```python
from build123d import *

# Parameters (mm, degrees)
F0_R     = 5.9319111077
F1_DEPTH = 114.3
F2_W     = 74.0328431129
F2_H     = 50.0019490719
F2_W_2   = 18.4651985765
F3_DEPTH = 30.2013677934
F4_DEPTH = 81.026


with BuildPart() as f1:
    # F0 (on Top) → F1 (new body)
    with BuildSketch(Plane.XY):
        with BuildLine():
            Line((15.1001838967, -37.0164215565), (15.1001838967, 37.0164215565))
            ThreePointArc((15.1001838967, 37.0164215565), (0, 21.9162376598), (-15.1001838967, 37.0164215565))
            Line((-15.1001838967, 37.0164215565), (-15.1001838967, -37.0164215565))
            ThreePointArc((-15.1001838967, -37.0164215565), (0, -21.9162376598), (15.1001838967, -37.0164215565))
        make_face()
        with BuildLine():
            ThreePointArc((-15.1001838967, -37.0164215565), (0, -52.1166054532), (15.1001838967, -37.0164215565))
            ThreePointArc((15.1001838967, -37.0164215565), (0, -21.9162376598), (-15.1001838967, -37.0164215565))
        make_face()
        with Locations((0, -37.0164215565)):
            Circle(F0_R, mode=Mode.SUBTRACT)
        with BuildLine():
            ThreePointArc((-15.1001838967, 37.0164215565), (0, 21.9162376598), (15.1001838967, 37.0164215565))
            ThreePointArc((15.1001838967, 37.0164215565), (0, 52.1166054532), (-15.1001838967, 37.0164215565))
        make_face()
        with Locations((0, 37.0164215565)):
            Circle(F0_R, mode=Mode.SUBTRACT)
    extrude(amount=F1_DEPTH)

    # F2 (on face) → F3 (cut, through all)
    with BuildSketch(Plane.YZ.offset(15.1001838967)):
        with Locations((0, 52.5265261531)):
            Rectangle(F2_W, F2_H)
        with Locations((-46.2490208447, 52.5265261531)):
            Rectangle(F2_W_2, F2_H)
        with Locations((46.2490208447, 52.5265261531)):
            Rectangle(F2_W_2, F2_H)
    extrude(amount=-F3_DEPTH, mode=Mode.SUBTRACT)

    # F0 (on Top) → F4 (join)
    with BuildSketch(Plane.XY):
        with BuildLine():
            ThreePointArc((-15.1001838967, 37.0164215565), (0, 21.9162376598), (15.1001838967, 37.0164215565))
            ThreePointArc((15.1001838967, 37.0164215565), (0, 52.1166054532), (-15.1001838967, 37.0164215565))
        make_face()
        with Locations((0, 37.0164215565)):
            Circle(F0_R, mode=Mode.SUBTRACT)
    extrude(amount=F4_DEPTH)


solid = f1.part
```
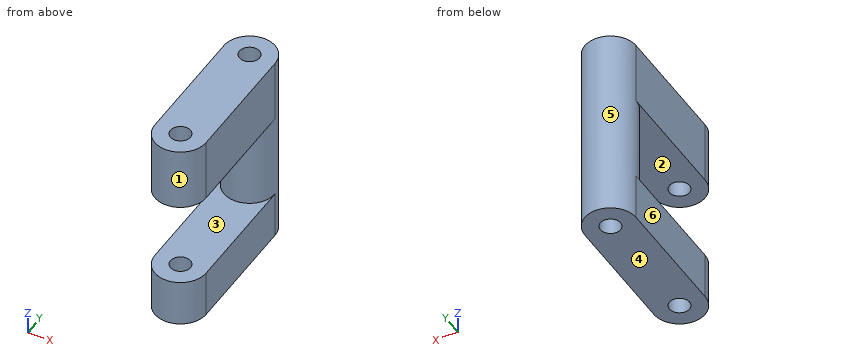
Build history of the part. All positions in model axes, mm. Face numbers are marked on the shaded views. A direction names the side the tool comes from. Give positions to 0.01 mm unless a question says otherwise; leave off trailing zeros. Loops run counter-clockwise (first coordinate to the right, second up) from the corner with the lowest first, then second, coordinate; pieces in that order, holes last.
Item 1: Slice it at A-A, the plane y = -6.5. List the corners of the cut face in (x, z).
Answers follow:
outline: (-15.1, 0) - (15.1, 0) - (15.1, 27.53) - (-15.1, 27.53) - close; (-15.1, 77.53) - (15.1, 77.53) - (15.1, 114.3) - (-15.1, 114.3) - close
Item 2: Which spindle directions (+Z, -Z, +X, -X, +Y, -Y) get a long thin tool onto all of the face, cutting with end or side? Do the marked faces 5 and 6. Say none if no direction does.
Answers follow:
face 5: none
face 6: +Z, -Z, -X, +Y, -Y
Item 3: Drill centre lines: line 1 (Y direction, x = 0, z = 19.75); line 2 (Y direction, x = 0, z = 37); line 3 (Z direction, x = -4, y = -9). Where is each one in solid material? Low to high.
Answers follow:
line 1: y = -52.12 to -42.95, -31.08 to 31.08, 42.95 to 52.12
line 2: y = 21.92 to 31.08, 42.95 to 52.12
line 3: z = 0 to 27.53, 77.53 to 114.3
Item 4: Slice it at D-D, the plane y = -45. List the corners of the cut face in (x, z).
Answers follow:
outline: (-12.82, 0) - (12.82, 0) - (12.82, 27.53) - (-12.82, 27.53) - close; (-12.82, 77.53) - (12.82, 77.53) - (12.82, 114.3) - (-12.82, 114.3) - close
Item 5: Slice it at B-B, the plane x = 0. List the corners of the cut face in (y, z).
Answers follow:
outline: (-52.12, 0) - (-42.95, 0) - (-42.95, 27.53) - (-52.12, 27.53) - close; (-52.12, 77.53) - (-42.95, 77.53) - (-42.95, 114.3) - (-52.12, 114.3) - close; (-31.08, 0) - (31.08, 0) - (31.08, 114.3) - (-31.08, 114.3) - (-31.08, 77.53) - (21.92, 77.53) - (21.92, 27.53) - (-31.08, 27.53) - close; (42.95, 0) - (52.12, 0) - (52.12, 114.3) - (42.95, 114.3) - close
Item 6: Flat gauge pins, fed straight in: pin 1 (10.5 mm diameter, centred on x = 0, y = 37.02, fed in from +Z); pin 2 (8 mm diameter, centred on y = -41.5, z = 98, fed in from -X); pin 3 (3 mm diameter, centred on x = -7.5, z = 16, fed in from +Y); pin 4 (6 mm diameter, centred on x = -9.5, z = 36, fed in from +Y). Where does each tip first touch, or does it go through?
Answers follow:
pin 1: passes through
pin 2: stops at x = -15.09
pin 3: stops at y = 50.87
pin 4: stops at y = 50.65
Item 7: Pull direction Z, two halves, no side cores. Call the marked faces 1, 2, 3 and 4: released by +Z, released by -Z, zero draft, split by the parting line, or undercut.
Answers follow:
face 1: zero draft
face 2: undercut
face 3: undercut
face 4: released by -Z
Item 8: Slice it at C-C, the plane z = 105. List the corners of the cut face in (x, y).
Answers follow:
outline: (-15.1, -37.02) arc R15.1 ccw to (15.1, -37.02) - (15.1, 37.02) arc R15.1 ccw to (-15.1, 37.02) - close; hole circle Ø11.86 at (0, -37.02); hole circle Ø11.86 at (0, 37.02)
